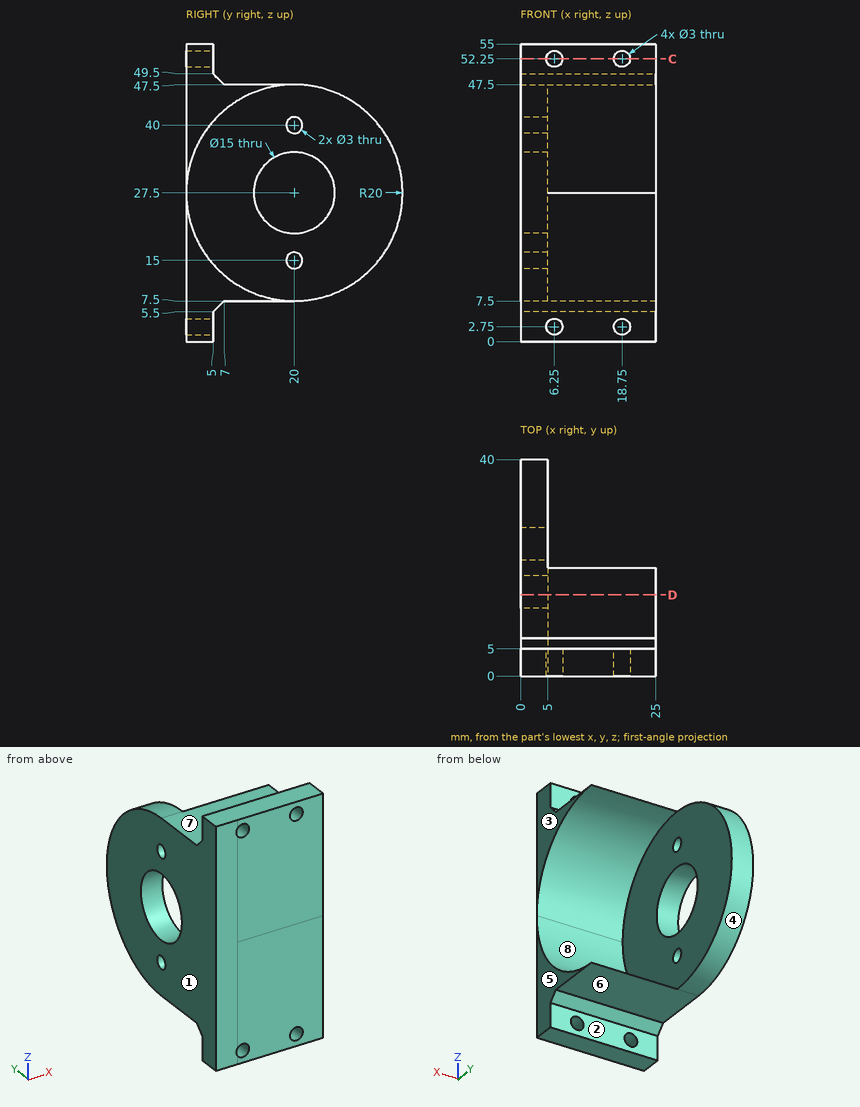
Design review of the part shown in the three views and the two pictorial views. Dimensions are in mm from the part's minimum x, y and z. A direction names the side the tool comes from. Give positions to 0.01 mm unless a question says otherwise; leave off trailing zeros. Write each loop counter-clockwise with the first axis right and the second up, starting at its lowest first coordinate (ties: lowest second). Pieces come first, ordered by that corner, then holes. Notation, with made-up numbers: M -27.75,47.25 L 0.25,47.25 A21 cw 0.25,60.25 Z; hole C 35,73.5 d1. An arc over 180 degrees is marked long. One line per question, with ' | ' between items. Start each with the question number.
Item 1: For pin 1 (2.5 mm diameter, centred on x = 18.75, z = 2.75, fed in from -Y); pin 2 (10.5 mm diameter, centred on x = 8, y = 15, fed in from +Z); pin 3 (6 mm diameter, centred on x = 12.5, z = 52, fed in from +Y); pin 4 (8 mm diameter, centred on y = 33, z = 30, fed in from +X), all flat-tipped, find the tip position at first contact; note any pin that passes through.
Item 2: We need section C-C on z = 52.25. Write out the cut boundary in (x, y).
Item 3: We need section D-D on y = 15. Write out the cut boundary in (x, z), plus the area to 3 significant figures.
Item 4: For the marked faces 4, 5, 6, 7 and 8, list the 3-axis set-ups (+Z, -Z, +X, -X, +Y, -Y) from which the entire face can be reached by the end or side of a thin tool; tool diameter is ignored.
Item 5: Wall thickness on line 1 (Z direction, x = 1, y = 20); line 2 (X direction, y = 3.25, z = 52.25); line 3 (Z direction, x = 18.75, y = 3.3) (3 decimals): over which ranges is each line inside the solid? List them lowest first. Write a range as from..to.
Item 6: Draft analysis for pull direction X (two halves, no side actions). For the marked faces 1, 2 and 3, state which applies: released by +X, released by -X, zero draft, split by the parting line, or undercut.
Results found:
1) pin 1: passes through | pin 2: stops at z = 47.5 | pin 3: stops at y = 5.5 | pin 4: stops at x = 5
2) outline: M 0,0 L 4.75,0 L 4.75,5 L 0,5 Z; M 7.75,0 L 17.25,0 L 17.25,5 L 7.75,5 Z; M 20.25,0 L 25,0 L 25,5 L 20.25,5 Z
3) outline: M 0,7.5 L 25,7.5 L 25,8.14 L 5,8.14 L 5,21.91 L 0,21.91 Z; M 0,33.09 L 5,33.09 L 5,46.86 L 25,46.86 L 25,47.5 L 0,47.5 Z | area: 170 mm2
4) face 4: +X, -X, +Y | face 5: +Z, -Z, +X, +Y, -Y | face 6: -Z, +X, -X, +Y | face 7: +Z, +X, -X, +Y | face 8: +X, +Y
5) line 1: z = 7.5..13.5, 16.5..20, 35..38.5, 41.5..47.5 | line 2: x = 0..4.75, 7.75..17.25, 20.25..25 | line 3: z = 0..1.25, 4.25..16.495, 38.505..50.75, 53.75..55
6) face 1: released by -X | face 2: zero draft | face 3: released by +X
